```python
from build123d import *

# Parameters (mm, degrees)
SKETCH1_W           = 352.425
SKETCH1_H           = 50.8
SKETCH1_R           = 9.525
SKETCH1_W_2         = 30.145810139
SKETCH1_H_2         = 23.882232645
BOSS_EXTRUDE1_DEPTH = 6.35
SKETCH2_R           = 1.776231012
CUT_EXTRUDE1_DEPTH  = 19.304


with BuildPart() as part:
    # Sketch1 → Boss-Extrude1 (new body)
    with BuildSketch(Plane.XY):
        with Locations((176.2125, 25.4)):
            Rectangle(SKETCH1_W, SKETCH1_H)
        with Locations((38.1, 25.4)):
            Circle(SKETCH1_R, mode=Mode.SUBTRACT)
        with Locations((314.325, 25.4)):
            Circle(SKETCH1_R, mode=Mode.SUBTRACT)
        with Locations((272.079290139, 23.364723209)):
            Rectangle(SKETCH1_W_2, SKETCH1_H_2, mode=Mode.SUBTRACT)
    extrude(amount=BOSS_EXTRUDE1_DEPTH)

    # Sketch2 → Cut-Extrude1 (cut)
    with BuildSketch(Plane.XZ):
        with Locations(Location((238.759223147, 3.175, 0), (0, 0, 270))):
            Circle(SKETCH2_R)
    extrude(amount=-CUT_EXTRUDE1_DEPTH, mode=Mode.SUBTRACT)


solid = part.part
```
Geometry check sheet. Reference: the model listing, model coordinates, mm. A direction names the side the tool comes from. Give positions to 0.01 mm unless a question says otherwise; leave off trailing zeros. Order: outer loops, then holes, each group sorted by start corner. A loop starts at its lowest first (then second) coordinate and runs counter-clockwise, first axis right, second up.
1. Access from +Z, -Z, +X, -X, +Y, -Y to the whole of each face (thin tool, end or side, straight path). Record for faces 1 (the face through (272, 35.306, 3)), 2 (the face through (0, 25, 3)).
2. Thickness scan on L1, parallel to X at y = 7, z = 3 (3 decimals); L2, parallel to Y at x = 268, z = 1.25; L3, parallel to Y at x = 38.1, z = 1.5 (3 decimals). Record the ranges inside material, lowest first.
3. Gauge pin test, flat end, axial feed: pin 1 Ø1.1 at (x, z) = (238.5, 4) entering from -Y. Record the tip position at first contact, or that the pin passes through.
4. Section check B-B, the plane x = 38.1. Enter the section's corners in (y, z) (3 decimals).
5. Release check for a two-part mould opening along X. For faces 3 (the face through (28.584, 25.819, 3.131)), 4 (the face through (174, 26, 0)), 5 (the face through (272, 11.424, 3)), 6 (the face through (352.425, 25, 3)) record: pulls with the +X half, pulls with the -X half, needs draft (parallel to the pull), parting line crosses it, or undercut.
6. Section check A-A, the plane y = 25.4. Enter the section's corners in (x, z) (3 decimals).
Values follow:
1. face 1: +Z, -Z
1. face 2: +Z, -Z, -X, +Y, -Y
2. L1: x = 0 to 236.992, 240.527 to 352.425
2. L2: y = 0 to 11.42, 35.31 to 50.8
2. L3: y = 0 to 15.875, 34.925 to 50.8
3. pin 1: stops at y = 19.3
4. outline: (0, 0) - (15.875, 0) - (15.875, 6.35) - (0, 6.35) - close; (34.925, 0) - (50.8, 0) - (50.8, 6.35) - (34.925, 6.35) - close
5. face 3: undercut
5. face 4: needs draft
5. face 5: undercut
5. face 6: pulls with the +X half
6. outline: (0, 0) - (28.575, 0) - (28.575, 6.35) - (0, 6.35) - close; (47.625, 0) - (257.006, 0) - (257.006, 6.35) - (47.625, 6.35) - close; (287.152, 0) - (304.8, 0) - (304.8, 6.35) - (287.152, 6.35) - close; (323.85, 0) - (352.425, 0) - (352.425, 6.35) - (323.85, 6.35) - close
